Work out the finished part from the listing and answer in its coordinate system (mm). A direction names the side the tool comes from. Coordinates: 2 decimals unless noted, no trailing zeros. Order: outer loops, then holes, each group sorted by start corner. A loop starts at its lowest first (then second) coordinate and runs counter-clockwise, first axis right, second up. Notation, with made-up numbers: (82.25, 39.25) -> (110.25, 39.25) arc R25 cw to (110.25, 55.25) -> close; hole circle Ø11 at (61.5, 42.5). An arc over 180 degrees is marked (long way). Use one line per item in the form item = value.
from build123d import *

# Parameters (mm, degrees)
SKETCH_2_W                   = 8
SKETCH_2_H                   = 24
EXTRUDE_1_DEPTH              = 10
SKETCH_3_W                   = 9.180468112
SKETCH_3_H                   = 14
CUT_EXTRUDE_1_DEPTH          = 40
CHAMFER_1_SIZE               = 1
HOLE_WIZARD_M3_1_D           = 3.2
HOLE_WIZARD_M3_1_CBORE_D     = 5.9
HOLE_WIZARD_M3_1_CBORE_DEPTH = 1.6
CUT_EXTRUDE_2_DEPTH          = 1.6
MM_2_D                       = 3
MM_2_DEPTH                   = 24
MM_2_TIP                     = 0.901290929
CHAMFER_2_SIZE               = 1


with BuildPart() as part:
    # 草图2 → 凸台-拉伸1 (new body)
    with BuildSketch(Plane.XY):
        with Locations((100, 93)):
            Rectangle(SKETCH_2_W, SKETCH_2_H)
    extrude(amount=EXTRUDE_1_DEPTH)

    # 草图3 → 切除-拉伸1 (cut)
    with BuildSketch(Plane.ZY.offset(-96)):
        with Locations((8.790234056, 93)):
            Rectangle(SKETCH_3_W, SKETCH_3_H)
    extrude(amount=-CUT_EXTRUDE_1_DEPTH, mode=Mode.SUBTRACT)

    # 倒角1
    chamfer_1_edges = [part.edges().sort_by_distance(p)[0] for p in [
        (100, 86, 4.2),
        (100, 100, 4.2),
    ]]
    chamfer(chamfer_1_edges, length=CHAMFER_1_SIZE)

    # M3 六角头螺栓的柱形沉头孔1 (through all)
    with Locations(Plane(origin=(124.363861944, -131.010130877, 4.2), x_dir=(0, 1, 0), z_dir=(0, 0, 1))):
        with Locations((221.010130877, 24.363861944), (227.010130877, 24.363861944)):
            CounterBoreHole(HOLE_WIZARD_M3_1_D / 2, HOLE_WIZARD_M3_1_CBORE_D / 2, HOLE_WIZARD_M3_1_CBORE_DEPTH)

    # 草图11 → 切除-拉伸2 (cut)
    with BuildSketch(Plane.XY.offset(4.2)):
        with BuildLine():
            Line((97.05, 90), (97.05, 96))
            ThreePointArc((97.05, 96), (100, 98.95), (102.95, 96))
            Line((102.95, 96), (102.95, 90))
            ThreePointArc((102.95, 90), (100, 87.05), (97.05, 90))
        make_face()
    extrude(amount=-CUT_EXTRUDE_2_DEPTH, mode=Mode.SUBTRACT)

    # 大小mm 暗销孔2
    with Locations(Plane(origin=(124.363861944, 105, -5), x_dir=(-1, 0, 0), z_dir=(0, 1, 0))):
        with Locations((24.363861944, 12.5)):
            Hole(MM_2_D / 2, depth=MM_2_DEPTH)
            with Locations((0, 0, -(MM_2_DEPTH + MM_2_TIP / 2))):  # 118° drill point
                Cone(0, MM_2_D / 2, MM_2_TIP, mode=Mode.SUBTRACT)

    # 倒角2
    chamfer_2_edges = [part.edges().sort_by_distance(p)[0] for p in [
        (96, 102.5, 10),
        (104, 102.5, 10),
        (96, 83.5, 10),
        (104, 83.5, 10),
    ]]
    chamfer(chamfer_2_edges, length=CHAMFER_2_SIZE)


solid = part.part
(1) Straight lines are drawn through the part: line 1 along Y through (x, z) = (100, 2.5); line 2 along X through (y, z) = (96, 1.8); line 3 along Z through (x, y) = (100, 103.8). For each, find the intervals that lie inside material, in ascending order.
Data:
line_1 = 81 to 88.4, 91.6 to 94.4, 97.6 to 105
line_2 = 96 to 98.4, 101.6 to 104
line_3 = 0 to 6, 9 to 10
(2) Section A-A on z = 7.5 is taken. Write down the section's boundary in (x, y), plus the area to 3 significant figures.
Data:
outline = (96, 81) -> (98.5, 81) -> (98.5, 86) -> (96, 86) -> close; (96, 100) -> (98.5, 100) -> (98.5, 105) -> (96, 105) -> close; (101.5, 81) -> (104, 81) -> (104, 86) -> (101.5, 86) -> close; (101.5, 100) -> (104, 100) -> (104, 105) -> (101.5, 105) -> close
area = 50.0 mm²
(3) The mould has two halves that part along Y. Classify faces 4 (the cylindrical face through (100.69, 83.46, 6.17)), 5 (the flat face through (99.9, 86.5, 4.7)): released by +Y, released by -Y, zero draft, split by the parting line, or undercut.
Data:
face_4 = zero draft
face_5 = undercut
(4) Section D-D on x = 100.75 is taken. Count the separate pieces of the cut face and the enclosed holes in it, plus the area to 3 significant figures.
Data:
separate_pieces = 5
enclosed_holes = 0
area = 100 mm²
(5) Section C-C on z = 2.25 is taken. Write down the section's boundary in (x, y).
Data:
outline = (96, 81) -> (104, 81) -> (104, 105) -> (96, 105) -> close; hole circle Ø3.2 at (100, 90); hole circle Ø3.2 at (100, 96)
(6) Each of these flat-tipped pins is pushed along its axis until it touches: P1, Ø2.5, axis at x = 100, z = 7.5, coming from the -Y side; P2, Ø4.5, axis at x = 100, y = 94.5, coming from the +Z side. Where does it stop, or does it pass through?
Data:
P1 = through
P2 = 2.6
(7) Section B-B on x = 96.75 is taken. Write down the section's boundary in (y, z).
Data:
outline = (81, 0) -> (105, 0) -> (105, 9.75) -> (100, 9.75) -> (100, 5.2) -> (99, 4.2) -> (87, 4.2) -> (86, 5.2) -> (86, 9.75) -> (81, 9.75) -> close
(8) Which of the six approach directions +Z, -Z, +X, -X, +Y, -Y give full straight-line access (tool end or side, diameter ignored) to faces 1 (the flat face through (99.9, 99.5, 4.7)), 2 (the flat face through (97.05, 93, 3)), 3 (the flat face through (100, 93, 0))?
Data:
face_1 = +Z, +X, -X
face_2 = +Z
face_3 = -Z, +X, -X, +Y, -Y
